Geometry check sheet. Reference: the model listing, model coordinates, mm. Face numbers are marked on the shaded views. A direction names the side the tool comes from. Coordinates: 2 decimals unless noted, no trailing zeros. Loops run counter-clockwise (first coordinate to the right, second up) from the corner with the lowest first, then second, coordinate; pieces in that order, holes last. Notation, with made-up numbers: (72, -36.5) -> (112, -36.5) arc R30 ccw to (112, -2.5) -> close; hole circle Ø10 at (67.5, 60.5). An arc over 180 degrees is marked (long way). Answer as a JSON object with one key per item and string values.
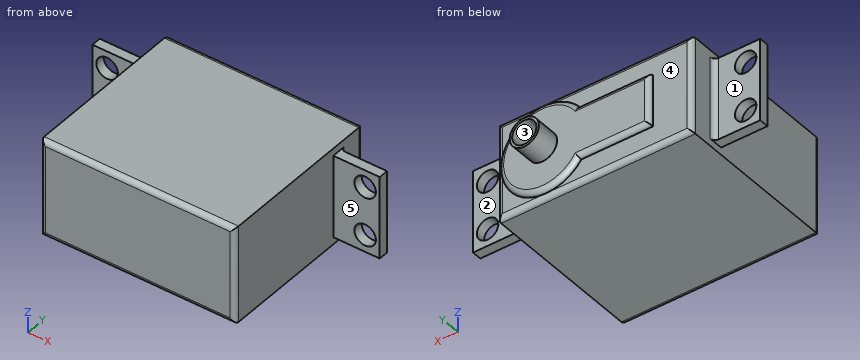
from build123d import *

# Parameters (mm, degrees)
SKETCH1_W           = 40
SKETCH1_H           = 35
BOSS_EXTRUDE1_DEPTH = 20
FILLET1_R           = 1
SKETCH2_W           = 9.556150209
SKETCH2_H           = 17
SKETCH2_R           = 2.209517665
BOSS_EXTRUDE2_DEPTH = 2
BOSS_EXTRUDE3_DEPTH = 1
SKETCH4_R           = 3
SKETCH4_R_2         = 2.5
BOSS_EXTRUDE4_DEPTH = 5
FILLET2_R           = 1


with BuildPart() as part:
    # Sketch1 → Boss-Extrude1 (new body)
    with BuildSketch(Plane.XY):
        Rectangle(SKETCH1_W, SKETCH1_H)
    extrude(amount=BOSS_EXTRUDE1_DEPTH)

    # Fillet1
    fillet1_edges = [part.edges().sort_by_distance(p)[0] for p in [
        (0, -17.5, 20),
        (0, -17.5, 0),
        (0, 17.5, 0),
        (20, -17.5, 10),
        (-20, -17.5, 10),
        (-20, 17.5, 10),
        (20, 17.5, 10),
        (0, 17.5, 20),
    ]]
    fillet(fillet1_edges, radius=FILLET1_R)

    # Sketch2 → Boss-Extrude2 (add)
    # profile 1 of 2: a face of its own
    with BuildSketch(Plane(origin=(0, 9.5, 0), x_dir=(-1, 0, 0), z_dir=(0, 1, 0))):
        with Locations((24.778075105, 10)):
            Rectangle(SKETCH2_W, SKETCH2_H)
        with Locations(Location((26.556150209, 5, 0), (0, 0, 270))):
            Circle(SKETCH2_R, mode=Mode.SUBTRACT)
        with Locations(Location((26.556150209, 15, 0), (0, 0, 90))):
            Circle(SKETCH2_R, mode=Mode.SUBTRACT)
    # profile 2 of 2: a face of its own
    with BuildSketch(Plane(origin=(0, 9.5, 0), x_dir=(-1, 0, 0), z_dir=(0, 1, 0))):
        with Locations((-24.778075105, 10)):
            Rectangle(SKETCH2_W, SKETCH2_H)
        with Locations(Location((-26.556150209, 5, 0), (0, 0, 90))):
            Circle(SKETCH2_R, mode=Mode.SUBTRACT)
        with Locations(Location((-26.556150209, 15, 0), (0, 0, 270))):
            Circle(SKETCH2_R, mode=Mode.SUBTRACT)
    extrude(amount=BOSS_EXTRUDE2_DEPTH)

    # Sketch3 → Boss-Extrude3 (add)
    with BuildSketch(Plane(origin=(0, 17.5, 0), x_dir=(1, 0, 0), z_dir=(0, 1, 0))):
        with BuildLine():
            Line((2.749933149, -4.667408636), (-12, -4.667408636))
            Line((-12, -4.667408636), (-12, -15.332591364))
            Line((-12, -15.332591364), (2.749933149, -15.332591364))
            ThreePointArc((2.749933149, -15.332591364), (19, -10), (2.749933149, -4.667408636))
        make_face()
    extrude(amount=BOSS_EXTRUDE3_DEPTH)

    # Sketch4 → Boss-Extrude4 (add)
    with BuildSketch(Plane(origin=(0, 18.5, 0), x_dir=(1, 0, 0), z_dir=(0, 1, 0))):
        with Locations(Location((10, -10, 0), (0, 0, 270))):
            Circle(SKETCH4_R)
        with Locations(Location((10, -10, 0), (0, 0, 270))):
            Circle(SKETCH4_R_2, mode=Mode.SUBTRACT)
    extrude(amount=BOSS_EXTRUDE4_DEPTH)

    # Fillet2
    fillet2_edges = [part.edges().sort_by_distance(p)[0] for p in [
        (20, 11.5, 10),
        (-20, 11.5, 10),
        (-12, 18.5, 10),
        (-4.625033426, 18.5, 4.667408636),
        (19, 18.5, 10),
        (-4.625033426, 18.5, 15.332591364),
    ]]
    fillet(fillet2_edges, radius=FILLET2_R - 0.0001)  # a hair under: the kernel refuses the full size


solid = part.part
1. Tool access check on the marked faces 1, 2, 3, 4 and 5. Record the directions out of +Z, -Z, +X, -X, +Y, -Y that give a thin tool (end or side, any length) a straight path to the whole face; none if there is none.
Evaluation:
{"face 1": "+Z, -Z, -X, +Y", "face 2": "+Z, -Z, +X, +Y", "face 3": "+Y", "face 4": "-X, +Y", "face 5": "+Z, -Z, +X, -Y"}
2. Section check A-A, the plane x = -25.5. Record the boundary of the cut face in (y, z).
Evaluation:
{"outline": "(9.5, 1.5) -> (11.5, 1.5) -> (11.5, 3.06) -> (9.5, 3.06) -> close; (9.5, 6.94) -> (11.5, 6.94) -> (11.5, 13.06) -> (9.5, 13.06) -> close; (9.5, 16.94) -> (11.5, 16.94) -> (11.5, 18.5) -> (9.5, 18.5) -> close"}
3. Thickness scan on probe 1 along X at (y, z) = (10.65, 5); probe 2 along Y at (x, z) = (-17.5, 8.75); probe 3 along Y at (x, z) = (10, 3.75). Record the ranges inside material, lowest first. Write a range as from..to.
Evaluation:
{"probe 1": "x = -29.56..-28.77, -24.35..24.35, 28.77..29.56", "probe 2": "y = -17.5..17.5", "probe 3": "y = -17.5..18.5"}
4. Depth check by flat-ended pin: P1, Ø1.5, axis at x = 25, y = 10.5, coming from the -Z side; P2, Ø3, axis at x = -18.5, z = 12.5, coming from the +Y side; P3, Ø5, axis at x = 23, z = 3.5, coming from the -Y side; P4, Ø3.5, axis at x = 26.56, z = 15, coming from the +Y side (3 decimals). Enter the tip coordinate at first touch or a pass-through.
Evaluation:
{"P1": "stops at z = 1.5", "P2": "stops at y = 17.5", "P3": "stops at y = 9.5", "P4": "passes through"}
5. Section check D-D, the plane x = -15. Record the boundary of the cut face in (y, z), then the cut area to 3 significant figures.
Evaluation:
{"outline": "(-17.5, 1) arc R1 ccw to (-16.5, 0) -> (16.5, 0) arc R1 ccw to (17.5, 1) -> (17.5, 19) arc R1 ccw to (16.5, 20) -> (-16.5, 20) arc R1 ccw to (-17.5, 19) -> close", "area": "699 mm^2"}
6. Section check C-C, the plane y = -5.5. Record the boundary of the cut face in (x, z), then the cut area to 3 significant figures.
Evaluation:
{"outline": "(-20, 0) -> (20, 0) -> (20, 20) -> (-20, 20) -> close", "area": "800 mm^2"}
